Check sheet for the drawn part. Datum: minimum x, y, z corner. Units: mm. A direction names the side the tool comes from. Round coordinates to 2 decimals unless told otherwise and drop trailing zeros. Write each loop counter-clockwise with the first axis right and the second up, starting at its lowest first coordinate (ties: lowest second). Pieces come first, ordered by that corner, then holes. Notation, with made-up numbers: M -14.75,33.5 L 11.25,33.5 A23 cw 11.25,43.5 Z; hole C -38,87 d2. An arc over 180 degrees is marked long. One line per item, written item: value. Start each with the question number.
Item 1: Section check D-D, the plane x = 21. Record the cut outline in (y, z).
Item 2: Thickness scan on probe 1 along Z at (x, y) = (29.9, 15.5); probe 2 along Z at (x, y) = (15, 2.5); probe 3 along X at (y, z) = (15.5, 10.7). Record the ranges inside material, lowest first. Write a range as from..to.
Item 3: Section check C-C, the plane z = 6. Record the cut outline in (x, y).
Item 4: Gauge pin test, flat ends, axial feed: pin 1 (1 mm diameter, centred on y = 9.5, z = 5.5, fed in from -X); pin 2 (1.5 mm diameter, centred on x = 16.5, z = 9.5, fed in from +Y); pin 3 (5 mm diameter, centred on y = 8.5, z = 7, fed in from +X). Record the tip position at first contact, or that the pin passes through.
Item 5: Section check A-A, the plane y = 15.5. Record the cut outline in (x, z), then the cut area to 3 significant figures.
Item 6: Tool access check on the marked faces 1 and 2. Record the directions out of +Z, -Z, +X, -X, +Y, -Y that give a thin tool (end or side, any length) a straight path to the whole face; none if there is none.
Item 7: Draft check along Y on the marked faces 3, 4 and 5. Enter one of: +Y half, -Y half, draft (parallel to the pull), parting line (faces both ways), or undercut.
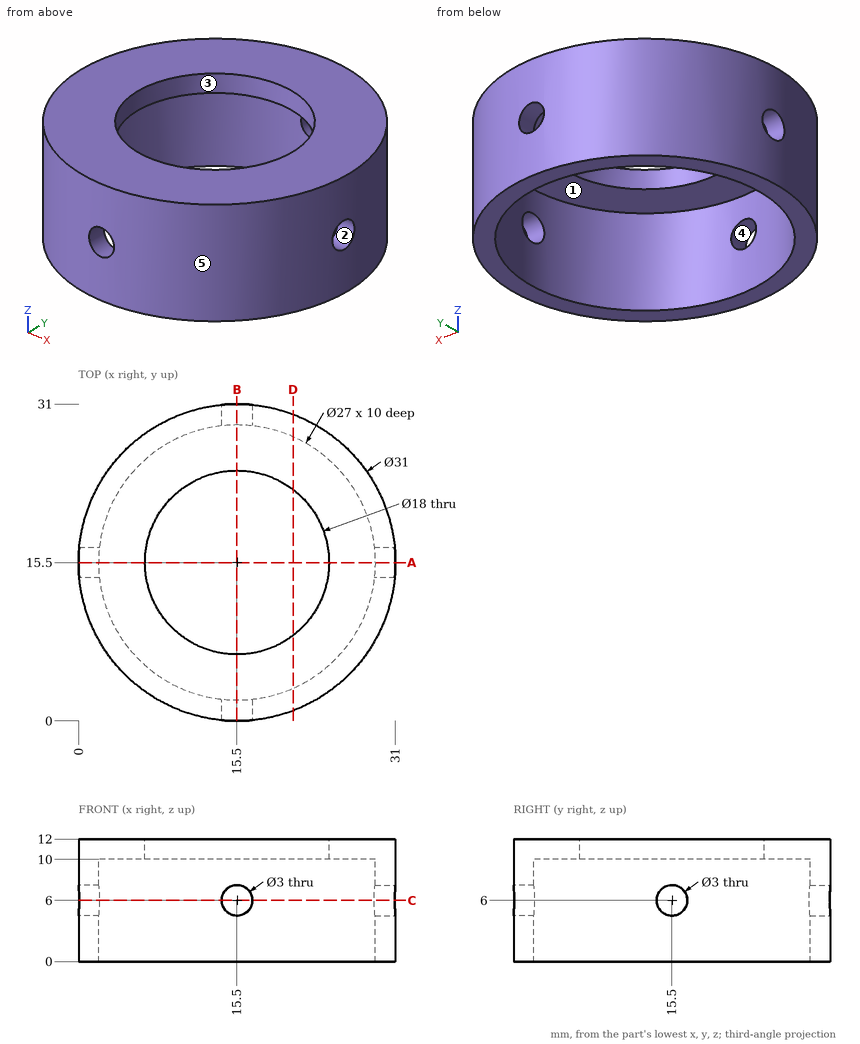
Response values:
1. outline: M 1.01,0 L 3.17,0 L 3.17,10 L 8.38,10 L 8.38,12 L 1.01,12 Z; M 22.62,10 L 27.83,10 L 27.83,0 L 29.99,0 L 29.99,12 L 22.62,12 Z
2. probe 1: z = 0..4.5, 7.5..12
2. probe 2: z = 10..12
2. probe 3: x = 0..6.5, 24.5..31
3. outline: M 0.07,14 A15.5 ccw 14,0.07 L 14,2.08 A13.5 cw 2.08,14 Z; M 0.07,17 L 2.08,17 A13.5 cw 14,28.92 L 14,30.93 A15.5 ccw Z; M 17,0.07 A15.5 ccw 30.93,14 L 28.92,14 A13.5 cw 17,2.08 Z; M 17,28.92 A13.5 cw 28.92,17 L 30.93,17 A15.5 ccw 17,30.93 Z
4. pin 1: stops at x = 1.01
4. pin 2: stops at y = 31
4. pin 3: stops at x = 30.33
5. outline: M 0,0 L 2,0 L 2,4.5 L 0,4.5 Z; M 0,7.5 L 2,7.5 L 2,10 L 6.5,10 L 6.5,12 L 0,12 Z; M 24.5,10 L 29,10 L 29,7.5 L 31,7.5 L 31,12 L 24.5,12 Z; M 29,0 L 31,0 L 31,4.5 L 29,4.5 Z
5. area: 54.0 mm2
6. face 1: -Z
6. face 2: +X, -X
7. face 3: undercut
7. face 4: draft
7. face 5: parting line
